```python
from build123d import *

# Parameters (mm, degrees)
BOSS_EXTRUDE1_DEPTH = 12.5
SKETCH15_R          = 1
BOSS_EXTRUDE2_DEPTH = 10
SKETCH19_R          = 0.625
CUT_EXTRUDE2_DEPTH  = 1
FILLET1_R           = 1
FILLET9_R           = 5
SKETCH32_W          = 30
SKETCH32_H          = 20
CUT_EXTRUDE10_DEPTH = 5
SKETCH34_R          = 0.625
CUT_EXTRUDE9_DEPTH  = 12.5


with BuildPart() as part:
    # Sketch1 → Boss-Extrude1 (new, symmetric)
    with BuildSketch(Plane.XY):
        with BuildLine():
            Line((-30, 2.5), (30, 2.5))
            Line((30, 2.5), (30, 0))
            add(Edge.make_bspline(
                [(-30, 0), (0, -7), (30, 0)],
                knots=[0, 0, 0, 1, 1, 1], degree=2))
            Line((-30, 0), (-30, 2.5))
        make_face()
        with BuildLine():
            Line((5, 7.5), (5, -3.402777778))
            Line((5, -3.402777778), (17.5, -7.5))
            Line((17.5, -7.5), (-17.5, -7.5))
            Line((-17.5, -7.5), (-5, -3.402777778))
            Line((-5, -3.402777778), (-5, 7.5))
            ThreePointArc((-5, 7.5), (0, 12.5), (5, 7.5))
        make_face()
    extrude(amount=BOSS_EXTRUDE1_DEPTH, both=True)

    # Sketch15 → Boss-Extrude2 (add)
    with BuildSketch(Plane(origin=(5, 0, 0), x_dir=(0, 0, -1), z_dir=(1, 0, 0))):
        with Locations((0, 5)):
            Circle(SKETCH15_R)
    boss_extrude2 = extrude(amount=BOSS_EXTRUDE2_DEPTH)

    # Sketch19 → Cut-Extrude2 (cut, symmetric)
    with BuildSketch(Plane.XY):
        with Locations((13, 5)):
            Circle(SKETCH19_R)
    cut_extrude2 = extrude(amount=CUT_EXTRUDE2_DEPTH, both=True, mode=Mode.SUBTRACT)

    # Mirror1: Boss-Extrude2, Cut-Extrude2 across plane
    add(boss_extrude2.mirror(Plane(origin=(0, 0, 0), x_dir=(0, 0, 1), z_dir=(1, 0, 0))))
    add(cut_extrude2.mirror(Plane(origin=(0, 0, 0), x_dir=(0, 0, 1), z_dir=(1, 0, 0))), mode=Mode.SUBTRACT)

    # Fillet1
    fillet1_edges = [part.edges().sort_by_distance(p)[0] for p in [
        (-30, 0, -6.25),
        (30, 0, 6.25),
        (5, 2.5, 0),
        (-5, 2.5, 0),
    ]]
    fillet(fillet1_edges, radius=FILLET1_R)

    # Fillet9
    # the kernel refuses this fillet: 5 mm, written as the material it adds along each edge
    with BuildSketch(Plane(origin=(5, -3.402777778, 12.5), x_dir=(0.9502551587034467, -0.3114725242416856, 0), z_dir=(0, 0, -1))) as fillet9_piece_1_section:
        with BuildLine():
            CenterArc((17.556244054, -2.371377478), FILLET9_R, 151.687811906, 90.630424807)
            Line((15.233443006, -6.799085157), (15.186986985, -6.88763931))
            ThreePointArc((15.186986985, -6.88763931), (7.684520329, -3.247724547), (-0.034816372, -0.093743374))
            Line((-0.034816372, -0.093743374), (0, 0.1))
            ThreePointArc((0, 0.1), (6.577180816, 0.1), (13.066323983, 0.04742755))
            Line((13.066323983, 0.04742755), (13.154361632, 0))
        make_face()
    fillet9_piece_1 = extrude(amount=12.5, mode=Mode.PRIVATE)
    fillet9_piece_1 = split(fillet9_piece_1, bisect_by=Plane(origin=(13.76615202, -7.5, 6.25), z_dir=(0, 1, 0)), keep=Keep.TOP, mode=Mode.PRIVATE)
    add(fillet9_piece_1)
    with BuildSketch(Plane(origin=(-5, -3.402777778, 0), x_dir=(-0.9946948021356532, 0.10287006660984462, 0), z_dir=(0, 0, 1))) as fillet9_piece_2_section:
        with BuildLine():
            CenterArc((16.998391443, 4.989972421), FILLET9_R, 175.740271774, 90.630424807)
            Line((12.012203504, 5.36136148), (11.912479745, 5.368789261))
            ThreePointArc((11.912479745, 5.368789261), (5.965344461, 2.771998007), (-0.040757291, 0.091317267))
            Line((-0.040757291, 0.091317267), (0.006413901, -0.099794097))
            ThreePointArc((0.006413901, -0.099794097), (8.340978482, 0.166269042), (16.675556633, -0.099799448))
            Line((16.675556633, -0.099799448), (16.681886727, 0))
        make_face()
    fillet9_piece_2 = extrude(amount=12.5, mode=Mode.PRIVATE)
    fillet9_piece_2 = split(fillet9_piece_2, bisect_by=Plane(origin=(-13.76615202, -7.5, 6.25), z_dir=(0, 1, 0)), keep=Keep.TOP, mode=Mode.PRIVATE)
    add(fillet9_piece_2)
    with BuildSketch(Plane(origin=(-5, -3.402777778, -12.5), x_dir=(-0.9502551587034468, -0.31147252424168526, 0), z_dir=(0, 0, 1))) as fillet9_piece_3_section:
        with BuildLine():
            CenterArc((17.556244054, -2.371377478), FILLET9_R, 151.687811906, 90.630424807)
            Line((15.233443006, -6.799085157), (15.186986985, -6.88763931))
            ThreePointArc((15.186986985, -6.88763931), (7.684520329, -3.247724547), (-0.034816372, -0.093743374))
            Line((-0.034816372, -0.093743374), (0, 0.1))
            ThreePointArc((0, 0.1), (6.577180816, 0.1), (13.066323983, 0.04742755))
            Line((13.066323983, 0.04742755), (13.154361632, 0))
        make_face()
    fillet9_piece_3 = extrude(amount=12.5, mode=Mode.PRIVATE)
    fillet9_piece_3 = split(fillet9_piece_3, bisect_by=Plane(origin=(-13.76615202, -7.5, -6.25), z_dir=(0, 1, 0)), keep=Keep.TOP, mode=Mode.PRIVATE)
    add(fillet9_piece_3)
    with BuildSketch(Plane(origin=(5, -3.402777778, 0), x_dir=(0.9502551587034467, -0.3114725242416856, 0), z_dir=(0, 0, -1))) as fillet9_piece_4_section:
        with BuildLine():
            CenterArc((17.556244054, -2.371377478), FILLET9_R, 151.687811906, 90.630424807)
            Line((15.233443006, -6.799085157), (15.186986985, -6.88763931))
            ThreePointArc((15.186986985, -6.88763931), (7.684520329, -3.247724547), (-0.034816372, -0.093743374))
            Line((-0.034816372, -0.093743374), (0, 0.1))
            ThreePointArc((0, 0.1), (6.577180816, 0.1), (13.066323983, 0.04742755))
            Line((13.066323983, 0.04742755), (13.154361632, 0))
        make_face()
    fillet9_piece_4 = extrude(amount=12.5, mode=Mode.PRIVATE)
    fillet9_piece_4 = split(fillet9_piece_4, bisect_by=Plane(origin=(13.76615202, -7.5, -6.25), z_dir=(0, 1, 0)), keep=Keep.TOP, mode=Mode.PRIVATE)
    add(fillet9_piece_4)

    # Sketch32 → Cut-Extrude10 (cut)
    with BuildSketch(Plane.XZ.offset(7.5)):
        Rectangle(SKETCH32_W, SKETCH32_H)
    extrude(amount=-CUT_EXTRUDE10_DEPTH, mode=Mode.SUBTRACT)

    # Sketch34 → Cut-Extrude9 (cut, symmetric)
    with BuildSketch(Plane.XY):
        with Locations((-8.75, -5)):
            Circle(SKETCH34_R)
        with Locations((8.75, -5)):
            Circle(SKETCH34_R)
    extrude(amount=CUT_EXTRUDE9_DEPTH, both=True, mode=Mode.SUBTRACT)


solid = part.part
```
Source: CAD feature listing. Evaluate the final solid. Frame: model axes, mm. A direction names the side the tool comes from. Coordinates: 2 decimals unless noted, no trailing zeros. Loops run counter-clockwise (first coordinate to the right, second up) from the corner with the lowest first, then second, coordinate; pieces in that order, holes last. Notation, with made-up numbers: M 63.5,14.25 L 76.5,14.25 A16 cw 76.5,28.25 Z; hole C -15,70 d11. An arc over 180 degrees is marked long. Put each result on its own line as item: value. Start each with the question number.
1) Cut plane B-B on x = -8.75. Return the cut outline in (y, z) (3 decimals), then the cut area to 3 significant figures.
2) Cut plane D-D on x = -1.5. Return the cut outline in (y, z), then the cut area to 3 significant figures.
3) Ray query, L1, parallel to X at y = 5, z = -0.1 (3 decimals); L2, parallel to Z at x = -0.5, y = -4.5; L3, parallel to Y at x = -13, z = -0.25 (3 decimals). Return the intervals inside material, ascending. Write a range as from..to.
4) Contact query for flat-ended pins moving along their axis: pin 1 Ø1.1 at (x, y) = (-13, 5) entering from -Z; pin 2 Ø1.2 at (y, z) = (5, 1) entering from +X; pin 3 Ø2 at (y, z) = (4.5, -0.5) entering from -X; pin 4 Ø2 at (y, z) = (5.5, 4) entering from -X. Output: stop coordinate, or through.
5) Reachability of faces 4 (the face through (15, 5, 0)), 5 (the face through (0, -2.5, 0)), 6 (the face through (-15, 5, 0)), 7 (the face through (10, 5, 1)) from +Z, -Z, +X, -X, +Y, -Y: full face, straight path, thin tool, end or side. Return the list, or none.
6) Cut plane C-C on y = -5. Return the cut outline in (x, z) (3 decimals).
7) Cut plane A-A on x = 7. Return the cut outline in (y, z).
8) Pull-direction query (Z, two-part tool) for faces 1 (the face through (0, 0, -12.5)), 2 (the face through (12.376, 5.027, 0.014)), 3 (the face through (0, -5, 10)); classes: pulls with the +Z half, pulls with the -Z half, needs draft (parallel to the pull), parting line crosses it, or undercut.
The answers:
1. outline: M -7.5,-12.5 L -5.625,-12.5 L -5.625,-10 L -7.5,-10 Z; M -7.5,10 L -5.625,10 L -5.625,12.5 L -7.5,12.5 Z; M -4.375,-12.5 L 2.5,-12.5 L 2.5,12.5 L -4.375,12.5 L -4.375,10 L -2.5,10 L -2.5,-10 L -4.375,-10 Z; C 5,0 d2
1. area: 147 mm²
2. outline: M -7.5,-12.5 L 12.27,-12.5 L 12.27,12.5 L -7.5,12.5 L -7.5,10 L -2.5,10 L -2.5,-10 L -7.5,-10 Z
2. area: 394 mm²
3. L1: x = -15..-13.625, -12.375..12.375, 13.625..15
3. L2: z = -12.5..-10, 10..12.5
3. L3: y = -2.5..2.5, 4.032..4.375, 5.625..5.968
4. pin 1: passes through
4. pin 2: stops at x = 15
4. pin 3: stops at x = -15
4. pin 4: stops at x = -5
5. face 4: +Z, -Z, +X, +Y
5. face 5: -Y
5. face 6: +Z, -Z, -X, +Y
5. face 7: +X
6. outline: M -17.69,-12.5 L -9.375,-12.5 L -9.375,-10 L -15,-10 L -15,10 L -9.375,10 L -9.375,12.5 L -17.69,12.5 Z; M -8.125,-12.5 L 8.125,-12.5 L 8.125,-10 L -8.125,-10 Z; M -8.125,10 L 8.125,10 L 8.125,12.5 L -8.125,12.5 Z; M 9.375,-12.5 L 17.69,-12.5 L 17.69,12.5 L 9.375,12.5 L 9.375,10 L 15,10 L 15,-10 L 9.375,-10 Z
7. outline: M -7.5,-12.5 L 2.5,-12.5 L 2.5,12.5 L -7.5,12.5 L -7.5,10 L -2.5,10 L -2.5,-10 L -7.5,-10 Z; C 5,0 d2
8. face 1: pulls with the -Z half
8. face 2: needs draft
8. face 3: undercut
